Autodesk Inventor part; units mm, degrees
ref_plane "YZ Plane" through (0, 0, 0) normal (1, 0, 0) x (0, 1, 0)
ref_plane "XZ Plane" through (0, 0, 0) normal (0, 1, 0) x (-1, 0, 0)
ref_plane "XY Plane" through (0, 0, 0) normal (0, 0, 1) x (1, 0, 0)
sketch "Skizze1" plane through (0, 0, 0) normal (0, 1, 0) x (-1, 0, 0)
  line L0 (35.5112, -88.3128) -> (35.5112, -108.3128)
  line L1 (35.5112, -108.3128) -> (22.0645, -123.1178)
  line L2 (22.0645, -123.1178) -> (2.0645, -123.1178)
  line L3 (2.0645, -123.1178) -> (-12.7404, -109.6711)
  line L4 (-12.7404, -109.6711) -> (-12.7404, -89.6711)
  line L5 (-12.7404, -89.6711) -> (0.7063, -74.8661)
  line L6 (0.7063, -74.8661) -> (20.7063, -74.8661)
  line L7 (20.7063, -74.8661) -> (35.5112, -88.3128)
  point P0 (0, 0)
  dimension "d0" = 20
  dimension "d1" = 20
  dimension "d2" = 20
  dimension "d3" = 20
  dimension "d4" = 20
  dimension "d5" = 20
  dimension "d6" = 20
  dimension "d7" = 20
extrude "Extrusion1" add sketch "Skizze1" along normal blind 3
sketch "Skizze2" plane through (-2.0645, 0, -123.1178) normal (0, 0, -1) x (-1, 0, 0)
  circle A0 centre (10, 1.5) radius 2.5
  line L0 (0, 3) -> (20, 3)
  point P0 (-2.0645, 0)
  dimension "d11" = 5
  dimension "d12" = 1.5
extrude "Extrusion2" add sketch "Skizze2" along normal blind 81.748
sketch "Skizze3" plane through (-12.0645, 1.5, -204.8658) normal (0, 0, -1) x (-1, 0, 0)
  line L0 (-35, -15) -> (35, -15)
  line L1 (35, -15) -> (35, 15)
  line L2 (35, 15) -> (-35, 15)
  line L3 (-35, 15) -> (-35, -15)
  arc A0 (2, -1.5) -> (-2, -1.5) centre (0, 0) ccw
  line L4 (-35, -15) -> (35, 15) construction
  line L5 (35, -15) -> (-35, 15) construction
  point P0 (-12.0645, -1.5)
  point P1 (-2, 1.5)
  point P2 (0, -2.5)
  point P3 (0, 2.5)
  dimension "d15" = 70
  dimension "d16" = 30
extrude "Extrusion3" add sketch "Skizze3" against normal blind 2
sketch "Skizze5" plane through (0, 0, 0) normal (0, -1, 0) x (1, 0, 0)
  line L0 (-22.0645, -123.1178) -> (51.5086, -123.1178)
  line L1 (51.5086, -123.1178) -> (51.5086, -51.2705)
  line L2 (51.5086, -51.2705) -> (-22.0645, -51.2705)
  line L3 (-22.0645, -51.2705) -> (-22.0645, -123.1178)
  line L4 (-22.0645, -51.2705) -> (-54.8687, -51.2705)
  line L5 (-54.8687, -51.2705) -> (-54.8687, -123.1178)
  line L6 (-54.8687, -123.1178) -> (-22.0645, -123.1178)
  line L7 (-22.0645, -123.1178) -> (-22.0645, -51.2705)
  point P0 (0, 0)
extrude "Extrusion5" cut sketch "Skizze5" against normal blind 10
properties part number "Stoppschild_Teil_Unten"
Check sheet for the modelled part. Datum: model origin and axes. Units: mm. A direction names the side the tool comes from. Round coordinates to 2 decimals unless told otherwise and drop trailing zeros. Write each loop counter-clockwise with the first axis right and the second up, starting at its lowest first coordinate (ties: lowest second). Pieces come first, ordered by that corner, then holes. Notation, with made-up numbers: (3.25, 71.25) - (7.25, 71.25) arc R15 ccw to (7.25, 100.25) - close; hole circle Ø3 at (32, 43.5). An arc over 180 degrees is marked (long way). Return JSON: item names as keys, results as strings.
Q1. Cross-section at C-C (z = -143). Record the boundary of the cut face in (x, y).
Returned:
{"outline": "circle Ø5 at (-12.06, 1.5)"}
Q2. Cross-section at A-A (y = 1.5). Record the boundary of the cut face in (x, z).
Returned:
{"outline": "(-47.06, -204.87) - (22.94, -204.87) - (22.94, -202.87) - (-9.56, -202.87) - (-9.56, -123.12) - (-14.56, -123.12) - (-14.56, -202.87) - (-47.06, -202.87) - close"}
Q3. Cross-section at B-B (x = 19). Record the boundary of the cut face in (y, z).
Returned:
{"outline": "(-13.5, -204.87) - (16.5, -204.87) - (16.5, -202.87) - (-13.5, -202.87) - close"}
Q4. Scan lines: L1, parallel to Z at x = 13, y = 6.25; L2, parallel to X at y = 3.5, z = -193.5; L3, parallel to Y at x = -13, z = -160. Record each from-to range of solid material in increasing order. Write a range as from..to.
Returned:
{"L1": "z = -204.87..-202.87", "L2": "x = -13.56..-10.56", "L3": "y = -0.82..3.82"}
Q5. Access from +Z, -Z, +X, -X, +Y, -Y to the whole of each face (thin tool, end or side, straight path). Record for faces 1 (the flat face through (-12, -13.5, -204)), 2 (the cylindrical face through (-9.567, 1.39, -162.434)).
Returned:
{"face 1": "+Z, -Z, +X, -X, -Y", "face 2": "+Z"}
Q6. Cross-section at D-D (y = -3.75). Record the boundary of the cut face in (x, z).
Returned:
{"outline": "(-47.06, -204.87) - (22.94, -204.87) - (22.94, -202.87) - (-47.06, -202.87) - close"}
Q7. Depth check by flat-ended pin: P1, Ø6, axis at y = 3, z = -172.5, coming from the +X side; P2, Ø6, axis at x = -15.5, z = -157.5, coming from the +Y side. Enter the tip coordinate at first touch or a pass-through.
Returned:
{"P1": "stops at x = -9.56", "P2": "stops at y = 3.96"}
